```python
from build123d import *

# Parameters (mm, degrees)
SKETCH1_R           = 4
BOSS_EXTRUDE1_DEPTH = 1.5
SKETCH2_R           = 2
CUT_EXTRUDE1_DEPTH  = 0.7
FILLET2_R           = 0.1
FILLET3_R           = 0.1


with BuildPart() as part:
    # Sketch1 → Boss-Extrude1 (new body)
    with BuildSketch(Plane(origin=(0, 0, 0), x_dir=(1, 0, 0), z_dir=(0, 1, 0))):
        Circle(SKETCH1_R)
    extrude(amount=BOSS_EXTRUDE1_DEPTH)

    # Sketch2 → Cut-Extrude1 (cut)
    with BuildSketch(Plane(origin=(0, 1.5, 0), x_dir=(1, 0, 0), z_dir=(0, 1, 0))):
        Circle(SKETCH2_R)
    extrude(amount=-CUT_EXTRUDE1_DEPTH, mode=Mode.SUBTRACT)

    # Fillet2
    fillet2_edges = [part.edges().sort_by_distance(p)[0] for p in [
        (-4, 0, 0),
    ]]
    fillet(fillet2_edges, radius=FILLET2_R)

    # Fillet3
    fillet3_edges = [part.edges().sort_by_distance(p)[0] for p in [
        (-4, 1.5, 0),
    ]]
    fillet(fillet3_edges, radius=FILLET3_R)


solid = part.part
```
The listing builds one solid part. Answer for the finished solid, in the listing's coordinates (mm). Round coordinates to 2 decimals unless told otherwise and drop trailing zeros. Order: outer loops, then holes, each group sorted by start corner. A loop starts at its lowest first (then second) coordinate and runs counter-clockwise, first axis right, second up. Notation, with made-up numbers: (4.25, -29.75) - (45.25, -29.75) arc R19 ccw to (45.25, -13.75) - close; hole circle Ø3 at (61, 32). An arc over 180 degrees is marked (long way). Put each result on its own line as item: value. Start each with the question number.
(1) Straight lines are drawn through the part: probe 1 along X at (y, z) = (1.15, 0); probe 2 along Y at (x, z) = (-0.5, -0.75). For each, find the intervals that lie inside material, in ascending order. Write a range as from..to.
(2) Find section C-C (y = 0.35). Give the vertices of the cut face in (x, z), plus the area to 3 significant figures.
(3) Find section A-A (x = 0). Give the vertices of the cut face in (y, z).
(4) Find section B-B (y = 1.05). Give the vertices of the cut face in (x, z), plus the area to 3 significant figures.
(5) Determine the mould class of faces 1 (the flat face through (0, 0.8, 0)), 2 (the cylindrical face through (0, 1, 2)), 3 (the cylindrical face through (-0.867, 0.741, 3.905)), 4 (the flat face through (-2, 1.5, -1)) for opening direction X: released by +X, released by -X, zero draft, split by the parting line, or undercut.
Reply:
1. probe 1: -4..-2, 2..4
1. probe 2: 0..0.8
2. outline: circle Ø8 at (0, 0)
2. area: 50.3 mm^2
3. outline: (0, -3.9) arc R0.1 ccw to (0.1, -4) - (1.4, -4) arc R0.1 ccw to (1.5, -3.9) - (1.5, -2) - (0.8, -2) - (0.8, 2) - (1.5, 2) - (1.5, 3.9) arc R0.1 ccw to (1.4, 4) - (0.1, 4) arc R0.1 ccw to (0, 3.9) - close
4. outline: circle Ø8 at (0, 0); hole circle Ø4 at (0, 0)
4. area: 37.7 mm^2
5. face 1: undercut
5. face 2: undercut
5. face 3: split by the parting line
5. face 4: zero draft
